```python
from build123d import *

# Parameters (mm, degrees)
CHAMFER3_SIZE = 2


with BuildPart() as part:
    # Sketch1 → Revolve1 (revolve)
    with BuildSketch(Plane(origin=(0, 0, 0), x_dir=(0, 0, -1), z_dir=(1, 0, 0))):
        Polygon((0, 0), (12, 0), (12, 26), (19, 26), (19, 29), (12, 29), (12, 129), (19, 129), (19, 132), (12, 132), (12, 184), (0, 184), align=None)
    revolve(axis=Axis((0, 184, 0), (0, -1, 0)))

    # Chamfer3
    chamfer3_edges = [part.edges().sort_by_distance(p)[0] for p in [
        (0, 0, 12),
        (0, 184, 12),
    ]]
    chamfer(chamfer3_edges, length=CHAMFER3_SIZE)


solid = part.part
```
Geometry: final body of the model. Coordinates: model frame, mm. A direction names the side the tool comes from. Round coordinates to 2 decimals unless told otherwise and drop trailing zeros. Write each loop counter-clockwise with the first axis right and the second up, starting at its lowest first coordinate (ties: lowest second). Pieces come first, ordered by that corner, then holes. Notation, with made-up numbers: (88.5, 11.5) -> (115.5, 11.5) arc R18 ccw to (115.5, 19.5) -> close; hole circle Ø10 at (49.25, 70.5). An arc over 180 degrees is marked (long way). Use CSV: the item, a comma, the result in double quotes. Start each with the question number.
Q1. Section D-D (y = 106). Return loops of the section in (x, z), plus the area to 3 significant figures.
Q2. Section A-A (x = 0). Return loops of the section in (y, z), plus the area to 3 significant figures.
Q3. Pull-direction query (Y, two-part tool) for faces 1 (the face through (-12.4, 26, -0.3)), 2 (the face through (-16.856, 27.521, -8.767)), 3 (the face through (0.53, 79.7, 11.99)); classes: pulls with the +Y half, pulls with the -Y half, needs draft (parallel to the pull), parting line crosses it, or undercut.
Q4. Section C-C (x = -15). Return loops of the section in (y, z), plus the area to 3 significant figures.
Q5. Reachability of faces 4 (the face through (0.53, 14.17, 11.99)), 5 (the face through (-12.4, 129, -0.3)), 6 (the face through (0.53, 157.35, 11.99)), 7 (the face through (-16.856, 130.521, -8.767)), 8 (the face through (0, 0, 0)) from +Z, -Z, +X, -X, +Y, -Y: full face, straight path, thin tool, end or side. Return the list, or none.
Q6. Section B-B (z = 0). Return loops of the section in (x, y).
Q7. First-contact query: pin 1 Ø1 at (x, y) = (10, 136) entering from +Z; pin 2 Ø10 at (x, z) = (-11.5, -14) entering from -Y; pin 3 Ø8 at (y, z) = (23, -13) entering from +X. Flat tips, straight axial feed; report the tip coordinate or a pass-through.
Q8. Line query: L1, parallel to Y at x = -12, z = 1; L2, parallel to Z at x = 9, y = 66.5; L3, parallel to Z at x = 10, y = 19.5. Output: solid intervals per line, ascending.
Result sheet:
1,outline,"circle Ø24 at (0, 0)"
1,area,"452 mm²"
2,outline,"(0, -10) -> (2, -12) -> (26, -12) -> (26, -19) -> (29, -19) -> (29, -12) -> (129, -12) -> (129, -19) -> (132, -19) -> (132, -12) -> (182, -12) -> (184, -10) -> (184, 10) -> (182, 12) -> (132, 12) -> (132, 19) -> (129, 19) -> (129, 12) -> (29, 12) -> (29, 19) -> (26, 19) -> (26, 12) -> (2, 12) -> (0, 10) -> close"
2,area,"4,490 mm²"
3,face 1,"pulls with the -Y half"
3,face 2,"needs draft"
3,face 3,"undercut"
4,outline,"(26, -11.66) -> (29, -11.66) -> (29, 11.66) -> (26, 11.66) -> close; (129, -11.66) -> (132, -11.66) -> (132, 11.66) -> (129, 11.66) -> close"
4,area,"140 mm²"
5,face 4,"-Y"
5,face 5,"none"
5,face 6,"+Y"
5,face 7,"+Y, -Y"
5,face 8,"+Z, -Z, +X, -X, -Y"
6,outline,"(-19, 26) -> (-12, 26) -> (-12, 2) -> (-10, 0) -> (10, 0) -> (12, 2) -> (12, 26) -> (19, 26) -> (19, 29) -> (12, 29) -> (12, 129) -> (19, 129) -> (19, 132) -> (12, 132) -> (12, 182) -> (10, 184) -> (-10, 184) -> (-12, 182) -> (-12, 132) -> (-19, 132) -> (-19, 129) -> (-12, 129) -> (-12, 29) -> (-19, 29) -> close"
7,pin 1,"z = 7.33"
7,pin 2,"y = 26"
7,pin 3,"x = 15.93"
8,L1,"26 to 29, 129 to 132"
8,L2,"-7.94 to 7.94"
8,L3,"-6.63 to 6.63"
